Input: dimensioned drawing with shaded views. Units: mm. Origin: part minimum x, y, z. Give positions to 0.01 mm unless a question says otherwise; leave off trailing zeros. Order: outer loops, then holes, each group sorted by start corner. A loop starts at its lowest first (then second) coordinate and runs counter-clockwise, first axis right, second up. Notation, with made-up numbers: M 10,50.25 L 20,50.25 A18 ccw 20,54.25 Z; hole C 58.25,-29 d2. An arc over 180 degrees is marked long. Answer in a Markdown table with one row per item. Add a question column.
(1) Pin query (flat end, axial travel): P1, Ø15, axis at y = 127, z = 12.7, coming from the -X side. Return the tip coordinate at first contact, or that it passes through.
(2) Section query C-C, the plane x = 35. Return loops of the section in (y, z) (1 decimal), plus the area to 3 significant figures.
(3) Mould query, pull axis X, two halves, no side actions, for the marked faces 1, 2 and 3. Classes: pulls with the +X half, pulls with the -X half, needs draft (parallel to the pull), parting line crosses it, or undercut.
(4) Section query A-A, the plane z = 12.7. Return loops of the section in (x, y), plus the area to 3 significant figures.
(5) Material intervals for line 1 along Y through (x, z) = (25, 12.5); line 2 along Z through (x, y) = (11, 12); line 3 along Z through (x, y) = (24, 127), sorted ascending.
(6) Section query B-B, the plane y = 12.7. Return loops of the section in (x, z), plus the area to 3 significant figures.
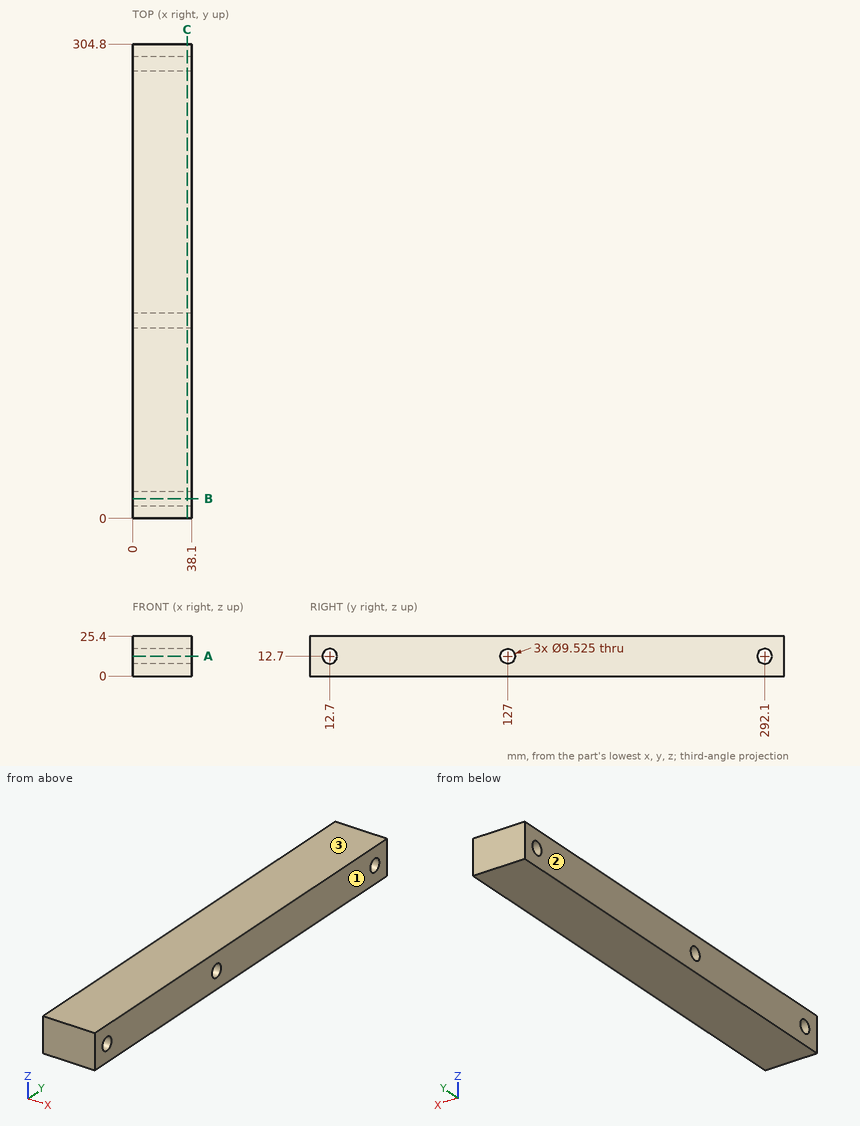
Values follow:
| question | item | result |
|---|---|---|
| 1 | P1 | stops at x = 0 |
| 2 | outline | M 0,0 L 304.8,0 L 304.8,25.4 L 0,25.4 Z; hole C 12.7,12.7 d9.5; hole C 127,12.7 d9.5; hole C 292.1,12.7 d9.5 |
| 2 | area | 7,530 mm² |
| 3 | face 1 | pulls with the +X half |
| 3 | face 2 | pulls with the -X half |
| 3 | face 3 | needs draft |
| 4 | outline | M 0,0 L 38.1,0 L 38.1,7.94 L 0,7.94 Z; M 0,17.46 L 38.1,17.46 L 38.1,122.24 L 0,122.24 Z; M 0,131.76 L 38.1,131.76 L 38.1,287.34 L 0,287.34 Z; M 0,296.86 L 38.1,296.86 L 38.1,304.8 L 0,304.8 Z |
| 4 | area | 10,500 mm² |
| 5 | line 1 | y = 0 to 7.94, 17.46 to 122.24, 131.76 to 287.34, 296.86 to 304.8 |
| 5 | line 2 | z = 0 to 7.99, 17.41 to 25.4 |
| 5 | line 3 | z = 0 to 7.94, 17.46 to 25.4 |
| 6 | outline | M 0,0 L 38.1,0 L 38.1,7.94 L 0,7.94 Z; M 0,17.46 L 38.1,17.46 L 38.1,25.4 L 0,25.4 Z |
| 6 | area | 605 mm² |
